from build123d import *

# Parameters (mm, degrees)
F0_W      = 38
F0_H      = 28.5
F1_DEPTH  = 19.5
F2_W      = 8
F2_H      = 15.5
F4_DEPTH  = 38
F6_DEPTH  = 19.5
F3_W      = 10
F3_H      = 9
F7_DEPTH  = 38
F9_DEPTH  = 38
F11_DEPTH = 7
F12_R     = 2
F13_DEPTH = 4
F15_DEPTH = 1.65
F17_DEPTH = 1.5
F19_DEPTH = 1.65
F21_DEPTH = 1.5
F23_DEPTH = 1.5
F25_DEPTH = 6
F27_DEPTH = 1.5
F29_DEPTH = 6
F30_W     = 38
F30_H     = 10.5
F31_DEPTH = 0.2
F33_DEPTH = 1.3
F34_R     = 1.25
F35_DEPTH = 4
F36_W     = 5.3
F36_H     = 2
F37_DEPTH = 8.65
F38_W     = 5.3
F38_H     = 2
F39_DEPTH = 8.65
F40_W     = 5.3
F40_H     = 2
F41_DEPTH = 5.15


with BuildPart() as f1:
    # F0 (on Top) → F1 (new body)
    with BuildSketch(Plane.XY):
        with Locations((3.11301895, 14.25)):
            Rectangle(F0_W, F0_H)
    extrude(amount=F1_DEPTH)

    # F2 (on face) → F4 (cut)
    with BuildSketch(Plane.YZ.offset(22.11301895)):
        with Locations((4, 11.75)):
            Rectangle(F2_W, F2_H)
    extrude(amount=-F4_DEPTH, mode=Mode.SUBTRACT)

    # F5 (on face) → F6 (cut)
    with BuildSketch(Plane.XY.offset(19.5)):
        with BuildLine():
            ThreePointArc((-8.4493121299, 27.5), (-11.38698105, 18.75), (-8.4493121299, 10))
            Line((-8.4493121299, 10), (14.6753500298, 10))
            ThreePointArc((14.6753500298, 10), (17.61301895, 18.75), (14.6753500298, 27.5))
            Line((14.6753500298, 27.5), (-8.4493121299, 27.5))
        make_face()
    extrude(amount=-F6_DEPTH, mode=Mode.SUBTRACT)

    # F3 (on face) → F7 (cut)
    with BuildSketch(Plane.YZ.offset(22.11301895)):
        with Locations((23.5, 15)):
            Rectangle(F3_W, F3_H)
    extrude(amount=-F7_DEPTH, mode=Mode.SUBTRACT)

    # F8 (on face) → F9 (cut)
    with BuildSketch(Plane.YZ.offset(22.11301895)):
        Polygon((18.5, 19.5), (8, 19.5), (8, 14), (10.5, 11.5), align=None)
    extrude(amount=-F9_DEPTH, mode=Mode.SUBTRACT)

    # F10 (on face) → F11 (cut)
    with BuildSketch(Plane(origin=(0, 0, 0), x_dir=(1, 0, 0), z_dir=(0, 0, -1))):
        with BuildLine():
            Line((15.5503619138, -9.5), (-9.3243240138, -9.5))
            ThreePointArc((-9.3243240138, -9.5), (-12.38698105, -18.75), (-9.3243240138, -28))
            Line((-9.3243240138, -28), (15.5503619138, -28))
            ThreePointArc((15.5503619138, -28), (18.61301895, -18.75), (15.5503619138, -9.5))
        make_face()
    extrude(amount=-F11_DEPTH, mode=Mode.SUBTRACT)

    # F12 (on face) → F13 (cut)
    with BuildSketch(Plane.XY.offset(4)):
        with Locations((-5.13698105, 4.25)):
            Circle(F12_R)
        with Locations((11.36301895, 4.25)):
            Circle(F12_R)
    extrude(amount=-F13_DEPTH, mode=Mode.SUBTRACT)

    # F14 (on face) → F15 (join)
    with BuildSketch(Plane.YZ.offset(22.11301895)):
        Polygon((8, 14), (10.5, 11.5), (18.5, 19.5), (16, 22), align=None)
    extrude(amount=-F15_DEPTH)

    # F16 (on face) → F17 (join)
    with BuildSketch(Plane(origin=(20.46301895, 0, 0), x_dir=(0, -1, 0), z_dir=(-1, 0, 0))):
        Polygon((-9.1564971157, 12.8435028843), (-8, 14), (-16, 22), (-17.1564971157, 20.8435028843), align=None)
    extrude(amount=F17_DEPTH)

    # F18 (on face) → F19 (join)
    with BuildSketch(Plane(origin=(-15.88698105, 0, 0), x_dir=(0, -1, 0), z_dir=(-1, 0, 0))):
        Polygon((-18.5, 19.5), (-10.5, 11.5), (-8, 14), (-16, 22), align=None)
    extrude(amount=-F19_DEPTH)

    # F20 (on face) → F21 (join)
    with BuildSketch(Plane.YZ.offset(-14.23698105)):
        Polygon((17.1564971157, 20.8435028843), (16, 22), (8, 14), (9.1564971157, 12.8435028843), align=None)
    extrude(amount=F21_DEPTH)

    # F22 (on face) → F23 (join)
    with BuildSketch(Plane(origin=(0, 9.5, 0), x_dir=(-1, 0, 0), z_dir=(0, 1, 0))):
        Polygon((-0.11301895, 3.8), (-3.11301895, 3.8), (-6.11301895, 3.8), (-6.11301895, 2.8), (-0.11301895, 2.8), align=None)
    extrude(amount=F23_DEPTH)

    # F24 (on face) → F25 (cut)
    with BuildSketch(Plane(origin=(0.11301895, 0, 0), x_dir=(0, -1, 0), z_dir=(-1, 0, 0))):
        Polygon((-11, 2.8), (-9.5, 2.8), (-11, 3.8), align=None)
    extrude(amount=-F25_DEPTH, mode=Mode.SUBTRACT)

    # F26 (on face) → F27 (join)
    with BuildSketch(Plane.XZ.offset(-28)):
        Polygon((6.11301895, 3.8), (3.11301895, 3.8), (0.11301895, 3.8), (0.11301895, 2.8), (6.11301895, 2.8), align=None)
    extrude(amount=F27_DEPTH)

    # F28 (on face) → F29 (cut)
    with BuildSketch(Plane(origin=(0.11301895, 0, 0), x_dir=(0, -1, 0), z_dir=(-1, 0, 0))):
        Polygon((-26.5, 3.8), (-28, 2.8), (-26.5, 2.8), align=None)
    extrude(amount=-F29_DEPTH, mode=Mode.SUBTRACT)

    # F30 (on face) → F31 (join)
    with BuildSketch(Plane(origin=(0, 28.5, 0), x_dir=(-1, 0, 0), z_dir=(0, 1, 0))):
        with Locations((-3.11301895, 5.25)):
            Rectangle(F30_W, F30_H)
    extrude(amount=F31_DEPTH)

    # F32 (on face) → F33 (cut)
    with BuildSketch(Plane(origin=(0, 0, 7), x_dir=(1, 0, 0), z_dir=(0, 0, -1))):
        with BuildLine():
            ThreePointArc((-9.0293473605, -9.5), (-9.4394942054, -10.4901820755), (-8.4493121299, -10.0800352306))
            Line((-8.4493121299, -10.0800352306), (-8.4493121299, -27.4199647694))
            ThreePointArc((-8.4493121299, -27.4199647694), (-9.4394942054, -27.0098179245), (-9.0293473605, -28))
            Line((-9.0293473605, -28), (15.2553852604, -28))
            ThreePointArc((15.2553852604, -28), (15.6655321053, -27.0098179245), (14.6753500298, -27.4199647694))
            Line((14.6753500298, -27.4199647694), (14.6753500298, -10.0800352306))
            ThreePointArc((14.6753500298, -10.0800352306), (15.6655321053, -10.4901820755), (15.2553852604, -9.5))
            Line((15.2553852604, -9.5), (-9.0293473605, -9.5))
        make_face()
    extrude(amount=-F33_DEPTH, mode=Mode.SUBTRACT)

    # F34 (on face) → F35 (cut)
    with BuildSketch(Plane(origin=(0, 0, 0), x_dir=(1, 0, 0), z_dir=(0, 0, -1))):
        with Locations((-9.88698105, -7)):
            Circle(F34_R)
        with Locations((16.11301895, -7)):
            Circle(F34_R)
        with Locations((3.11301895, -2.5)):
            Circle(F34_R)
    extrude(amount=-F35_DEPTH, mode=Mode.SUBTRACT)

    # F36 (on face) → F37 (cut)
    with BuildSketch(Plane(origin=(-15.88698105, 0, 0), x_dir=(0, -1, 0), z_dir=(-1, 0, 0))):
        with Locations((-7, 1)):
            Rectangle(F36_W, F36_H)
    extrude(amount=-F37_DEPTH, mode=Mode.SUBTRACT)

    # F38 (on face) → F39 (cut)
    with BuildSketch(Plane.YZ.offset(22.11301895)):
        with Locations((7, 1)):
            Rectangle(F38_W, F38_H)
    extrude(amount=-F39_DEPTH, mode=Mode.SUBTRACT)

    # F40 (on face) → F41 (cut)
    with BuildSketch(Plane.XZ):
        with Locations((3.11301895, 1)):
            Rectangle(F40_W, F40_H)
    extrude(amount=-F41_DEPTH, mode=Mode.SUBTRACT)


solid = f1.part
Build history of the part. All positions in model axes, mm. A direction names the side the tool comes from. Coordinates: 2 decimals unless noted, no trailing zeros. Order: outer loops, then holes, each group sorted by start corner. A loop starts at its lowest first (then second) coordinate and runs counter-clockwise, first axis right, second up. Notation, with made-up numbers: M 3,-19.5 L 41,-19.5 A35 ccw 41,15.5 Z; hole C -20.5,25.25 d4. An arc over 180 degrees is marked long. One line per question, with ' | ' between items. Start each with the question number.
Q1. Saw through at B-B (x = -2). List the corners of the cut face in (y, z).
Q2. Flat gauge pins, fed straight in: pin 1 Ø2 at (x, y) = (-0.5, 9.5) entering from +Z; pin 2 Ø3 at (x, y) = (-5.14, 4.25) entering from +Z; pin 3 Ø0.9 at (x, y) = (8, 27.5) entering from -Z; pin 4 Ø5 at (x, z) = (7.5, 15) entering from +Y. Where does each tip first touch, or does it go through?
Q3. Two-plate mould, pull along Z, no slides. Class faces 6 (the face through (-9.605, 27.348, 7.641)), 7 (the face through (20.463, 14, 16)), 8 (the face through (21, 17, 21)): +Z half, -Z half, draft (parallel to the pull), parting line (faces both ways), or undercut.
Q4. Saw through at C-C (y = 14.5). List the corners of the cut face in (x, z).
Q5. Probe L1, parallel to X at y = 9.75, z = 15; L2, parallel to Y at x = -6, z = 7; L3, parallel to X at y = 7.5, z = 2.5. List the from-to ranges inside material, lowest first. Write a range as from..to.
Q6. Saw through at D-D (z = 6). List the corners of the cut face in (x, y), then the cut area to 3 significant figures.
Q7. 3-axis set-ups, long thin cutter, end or side, ignore diameter. For faces 1 (the face through (18, 7, 2)), 2 (the face through (3, 5.15, 1)), 3 (the face through (3, 10, 3.8)), 4 (the face through (-12, 7, 2)), 5 (the face through (17.444, 16.54, 10.56)): which of +Z, -Z, +X, -X, +Y, -Y reach the whole face in a straight line?
Q8. Saw through at A-A (z = 9). List the corners of the cut face in (x, y), then the cut area to 3 significant figures.
Check values:
1) outline: M 0,0 L 9.5,0 L 9.5,8.3 L 10,8.3 L 10,12 L 8,14 L 8,4 L 0,4 Z; M 27.5,8.3 L 28,8.3 L 28,0 L 28.7,0 L 28.7,10.5 L 27.5,10.5 Z
2) pin 1: stops at z = 13.5 | pin 2: passes through | pin 3: stops at z = 8.3 | pin 4: stops at y = 9.5
3) face 6: draft | face 7: undercut | face 8: +Z half
4) outline: M -15.89,0 L -11.79,0 L -11.79,7 L -10.75,7 L -10.75,15.5 L -14.24,15.5 L -14.24,18.19 L -12.74,18.19 L -12.74,20.5 L -15.89,20.5 Z; M 16.98,7 L 18.02,7 L 18.02,0 L 22.11,0 L 22.11,20.5 L 18.96,20.5 L 18.96,18.19 L 20.46,18.19 L 20.46,15.5 L 16.98,15.5 Z
5) L1: x = -15.89..-12.74, 18.96..22.11 | L2: y = 8..9.5, 28..28.7 | L3: x = -15.89..-11.03, -8.74..14.97, 17.26..22.11
6) outline: M -15.89,8 L 22.11,8 L 22.11,28.7 L -15.89,28.7 Z; hole M -9.32,9.5 L 15.55,9.5 A15.5 ccw 15.55,28 L -9.32,28 A15.5 ccw Z | area: 249 mm2
7) face 1: -Z, +X | face 2: -Z, -Y | face 3: none | face 4: -Z, -X | face 5: +Z, -Z
8) outline: M -15.89,8 L 22.11,8 L 22.11,28.7 L -15.89,28.7 Z; hole M -8.45,10 L 14.68,10 A14.5 ccw 14.68,27.5 L -8.45,27.5 A14.5 ccw Z | area: 312 mm2
